Geometry: final body of the model. Coordinates: model frame, mm. Face numbers are marked on the shaded views. A direction names the side the tool comes from. Coordinates: 2 decimals unless noted, no trailing zeros. Order: outer loops, then holes, each group sorted by start corner. A loop starts at its lowest first (then second) coordinate and runs counter-clockwise, first axis right, second up. Notation, with made-up numbers: (-36.75, 20) -> (-16.75, 20) arc R15 ccw to (-16.75, 44) -> close; hole circle Ø8 at (-20.75, -38). An arc over 180 degrees is marked (long way). Answer in a Markdown table with one row per item. Add a question column.
1) Ray query, line 1 (Y direction, x = 1.5, z = 5.25); line 2 (Z direction, x = 10, y = -4.5). Return the intervals inside material, ascending. Write a range as from..to.
2) Contact query for a flat-ended pin moving along its axis: P1, Ø1.1, axis at x = 1.5, y = -5, coming from the -Z side. Output: stop coordinate, or through.
3) Section query B-B on y = -5. Return the cut outline in (x, z), then the cut area to 3 significant figures.
4) Set-up query: the marked faces 1 and 2. Return all of +Z, -Z, +X, -X, +Y, -Y with unobstructed straight access to the full face (end or side cutting, diameter ignored); none if empty.
5) Section query A-A on x = 6. Return the cut outline in (y, z), then the cut area to 4 significant figures.
6) Section query D-D on y = -8.5. Return the cut outline in (x, z), then the cut area to 3 significant figures.
7) Section query C-C on x = 1.5. Return the cut outline in (y, z).
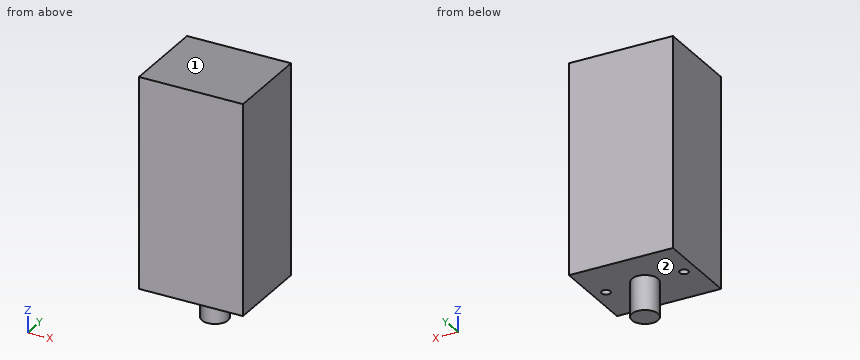
```python
from build123d import *

# Parameters (mm, degrees)
SKETCH1_W           = 12
SKETCH1_H           = 10
BOSS_EXTRUDE1_DEPTH = 24.25
SKETCH2_R           = 0.5
CUT_EXTRUDE1_DEPTH  = 10
SKETCH3_R           = 1.5
BOSS_EXTRUDE2_DEPTH = 4


with BuildPart() as part:
    # Sketch1 → Boss-Extrude1 (new body)
    with BuildSketch(Plane.XY):
        with Locations((6, -5)):
            Rectangle(SKETCH1_W, SKETCH1_H)
    extrude(amount=BOSS_EXTRUDE1_DEPTH)

    # Sketch2 → Cut-Extrude1 (cut)
    with BuildSketch(Plane(origin=(0, 0, 0), x_dir=(-1, 0, 0), z_dir=(0, 0, -1))):
        with Locations((-10.5, -5)):
            Circle(SKETCH2_R)
        with Locations((-1.5, -5)):
            Circle(SKETCH2_R)
    extrude(amount=-CUT_EXTRUDE1_DEPTH, mode=Mode.SUBTRACT)

    # Sketch3 → Boss-Extrude2 (add)
    with BuildSketch(Plane(origin=(0, 0, 0), x_dir=(-1, 0, 0), z_dir=(0, 0, -1))):
        with Locations(Location((-6, -5, 0), (0, 0, 180))):
            Circle(SKETCH3_R)
    extrude(amount=BOSS_EXTRUDE2_DEPTH)


solid = part.part
```
Result:
| question | item | result |
|---|---|---|
| 1 | line 1 | -10..-5.5, -4.5..0 |
| 1 | line 2 | 0..24.25 |
| 2 | P1 | z = 0 |
| 3 | outline | (0, 0) -> (1, 0) -> (1, 10) -> (2, 10) -> (2, 0) -> (4.5, 0) -> (4.5, -4) -> (7.5, -4) -> (7.5, 0) -> (10, 0) -> (10, 10) -> (11, 10) -> (11, 0) -> (12, 0) -> (12, 24.25) -> (0, 24.25) -> close |
| 3 | area | 283 mm2 |
| 4 | face 1 | +Z, +X, -X, +Y, -Y |
| 4 | face 2 | -Z |
| 5 | outline | (-10, 0) -> (-6.5, 0) -> (-6.5, -4) -> (-3.5, -4) -> (-3.5, 0) -> (0, 0) -> (0, 24.25) -> (-10, 24.25) -> close |
| 5 | area | 254.5 mm2 |
| 6 | outline | (0, 0) -> (12, 0) -> (12, 24.25) -> (0, 24.25) -> close |
| 6 | area | 291 mm2 |
| 7 | outline | (-10, 0) -> (-5.5, 0) -> (-5.5, 10) -> (-4.5, 10) -> (-4.5, 0) -> (0, 0) -> (0, 24.25) -> (-10, 24.25) -> close |
